Can you work these out from the model? Positions are in its coordinate system, mm. A direction names the side the tool comes from. Coordinates: 2 decimals unless noted, no trailing zeros. Order: outer loops, then holes, each group sorted by start corner. A loop starts at its lowest first (then second) coordinate and runs counter-clockwise, first axis right, second up. Notation, with made-up numbers: (-38.5, 16) -> (4.5, 16) arc R10 ccw to (4.5, 23) -> close; hole circle Ø9 at (18, 6). An arc over 180 degrees is marked (long way). Answer in a Markdown table with one row per item.
```python
from build123d import *

# Parameters (mm, degrees)
F0_W     = 38.1
F0_H     = 25.4
F1_DEPTH = 12.7
F2_W     = 21.2713289022
F2_H     = 12.695313897
F3_DEPTH = 25.4
F4_W     = 25.6905510694
F4_H     = 6.4952769317
F5_DEPTH = 24.13


with BuildPart() as f1:
    # F0 (on Front) → F1 (new body, symmetric)
    with BuildSketch(Plane.XZ):
        with Locations((19.05, 12.7)):
            Rectangle(F0_W, F0_H)
    extrude(amount=F1_DEPTH, both=True)

    # F2 (on face) → F3 (cut)
    with BuildSketch(Plane.XY.offset(25.4)):
        with Locations((27.4643355489, -0.1476199832)):
            Rectangle(F2_W, F2_H)
    extrude(amount=-F3_DEPTH, mode=Mode.SUBTRACT)

    # F4 (on face) → F5 (join)
    with BuildSketch(Plane.YZ.offset(38.1)):
        with Locations((-0.1452755347, 3.2476384658)):
            Rectangle(F4_W, F4_H)
    extrude(amount=-F5_DEPTH)


solid = f1.part
```
(1) Suppose I cut it at C-C (y = 4). Please give me the cut outline in (x, z), and give its area (3 significant figures).
Response values:
| item | result |
|---|---|
| outline | (0, 0) -> (38.1, 0) -> (38.1, 6.5) -> (16.83, 6.5) -> (16.83, 25.4) -> (0, 25.4) -> close |
| area | 566 mm2 |
(2) On a 3-axis mill with a long thin cutter (end or side, diameter ignored), from which of +Z, -Z, +X, -X, +Y, -Y can I reach the whole of each face in a straight line? I mean faces 1 (the flat face through (27, -6.495, 16)), 2 (the flat face through (0, 0, 13)). Say none if no direction works.
Response values:
| item | result |
|---|---|
| face 1 | +Z, +X |
| face 2 | +Z, -Z, -X, +Y, -Y |
(3) Suppose I cut it at B-B (z = 9.5). Please give me the cut outline in (x, y), and give its area (3 significant figures).
Response values:
| item | result |
|---|---|
| outline | (0, -12.7) -> (38.1, -12.7) -> (38.1, -6.5) -> (16.83, -6.5) -> (16.83, 6.2) -> (38.1, 6.2) -> (38.1, 12.7) -> (0, 12.7) -> close |
| area | 698 mm2 |
(4) Will these pins go through, and if not, where does the flat tip stop? pin 1 Ø3 at (y, z) = (1, 20) entering from +X; pin 2 Ø5.5 at (x, z) = (25.5, 16.5) entering from -Y; pin 3 Ø14 at (y, z) = (2.5, 16) entering from +X; pin 4 Ø4 at (x, y) = (22.5, 0) entering from +Z.
Response values:
| item | result |
|---|---|
| pin 1 | x = 16.83 |
| pin 2 | y = -12.7 |
| pin 3 | x = 38.1 |
| pin 4 | z = 6.5 |
(5) Suppose I cut it at A-A (x = 30). Please give me the cut outline in (y, z), and give its area (3 significant figures).
Response values:
| item | result |
|---|---|
| outline | (-12.99, 0) -> (12.7, 0) -> (12.7, 25.4) -> (6.2, 25.4) -> (6.2, 6.5) -> (-6.5, 6.5) -> (-6.5, 25.4) -> (-12.7, 25.4) -> (-12.7, 6.5) -> (-12.99, 6.5) -> close |
| area | 407 mm2 |
(6) I need wall thicknesses on line 1 (Y direction, x = 21, z = 16); line 2 (X direction, y = -0.5, z = 8.75); line 3 (Y direction, x = 12.5, z = 10.5). Which ranges of each line are inside material? Lowest first, please. Write a range as [from, to].
Response values:
| item | result |
|---|---|
| line 1 | [-12.7, -6.5], [6.2, 12.7] |
| line 2 | [0, 16.83] |
| line 3 | [-12.7, 12.7] |
(7) We'd pull the mould along Y, two halves only. Please class faces 3 (the flat face through (16.829, 0, 16)), 4 (the flat face through (26, -12.991, 3)), 5 (the flat face through (38.1, 0, 4)): +Y half, -Y half, draft (parallel to the pull), parting line (faces both ways), or undercut.
Response values:
| item | result |
|---|---|
| face 3 | undercut |
| face 4 | -Y half |
| face 5 | draft |
